from build123d import *

# Parameters (mm, degrees)
F0_R     = 11.25
F1_DEPTH = 3
F2_R     = 9.5
F3_DEPTH = 7.5
F4_R     = 3.75
F5_DEPTH = 7.5
F6_R     = 0.25
F7_DEPTH = 6
F8_SIZE2 = 0.288675
F8_SIZE  = 0.5
F9_R     = 0.3
F10_R    = 2.5


with BuildPart() as f1:
    # F0 (on Top) → F1 (new body)
    with BuildSketch(Plane.XY):
        Circle(F0_R)
    extrude(amount=F1_DEPTH)

    # F2 (on Top) → F3 (join)
    with BuildSketch(Plane.XY):
        Circle(F2_R)
    extrude(amount=F3_DEPTH)

    # F4 (on Top) → F5 (join)
    with BuildSketch(Plane.XY):
        Circle(F4_R)
    extrude(amount=-F5_DEPTH)

    # F6 (on Top) → F7 (join)
    with BuildSketch(Plane.XY):
        with Locations((0, 3.75)):
            Circle(F6_R)
        with Locations((3.75, 0)):
            Circle(F6_R)
        with Locations((0, -3.75)):
            Circle(F6_R)
        with Locations((-3.75, 0)):
            Circle(F6_R)
    extrude(amount=-F7_DEPTH)

    # F8
    f8_edges = [f1.edges().sort_by_distance(p)[0] for p in [
        (-3.75, 0, -7.5),
    ]]
    chamfer(f8_edges, length=F8_SIZE, length2=F8_SIZE2)

    # F9
    f9_edges = [f1.edges().sort_by_distance(p)[0] for p in [
        (-11.25, 0, 3),
    ]]
    fillet(f9_edges, radius=F9_R)

    # F10
    f10_edges = [f1.edges().sort_by_distance(p)[0] for p in [
        (-9.5, 0, 7.5),
    ]]
    fillet(f10_edges, radius=F10_R)


solid = f1.part
Verification items for the finished model (mm, model axes). A direction names the side the tool comes from. Coordinates: 2 decimals unless noted, no trailing zeros. Write each loop counter-clockwise with the first axis right and the second up, starting at its lowest first coordinate (ties: lowest second). Pieces come first, ordered by that corner, then holes. Notation, with made-up numbers: (-14, 53) - (22, 53) arc R24 ccw to (22, 74) - close; hole circle Ø11 at (-2.5, -7.75). An arc over 180 degrees is marked (long way). Answer as a JSON object with one key per item and string values.
(1) Mould release check, pull along Y, two halves, no side actions. Record for faces 4 (the cylindrical face through (3.464, -1.436, -3.451)), 5 (the flat face through (0, 0, -7.5)): pulls with the +Y half, pulls with the -Y half, needs draft (parallel to the pull), parting line crosses it, or undercut.
Report:
{"face 4": "parting line crosses it", "face 5": "needs draft"}
(2) Thickness scan on line 1 along Z through (x, y) = (-3.25, 9.25); line 2 along Z through (x, y) = (-1.25, 5); line 3 along X through (y, z) = (0.5, -3.75). Record the ranges inside material, lowest first.
Report:
{"line 1": "0 to 3", "line 2": "0 to 7.5", "line 3": "-3.72 to 3.72"}
(3) Tool access check on faces 1 (the flat face through (0, 10, 3)), 2 (the cylindrical face through (5.19, -9.98, 1.33)), 3 (the flat face through (-3, 3, 0)). Record the directions out of +Z, -Z, +X, -X, +Y, -Y that give a thin tool (end or side, any length) a straight path to the whole face; none if there is none.
Report:
{"face 1": "+Z", "face 2": "+Z, -Z", "face 3": "-Z"}
(4) Gauge pin test, flat ends, axial feed: pin 1 Ø1.5 at (y, z) = (5, 4.5) entering from +X; pin 2 Ø8 at (x, z) = (-4, -5.5) entering from +Y; pin 3 Ø4 at (y, z) = (-3.5, 1) entering from +X. Record the tip position at first contact, or that the pin passes through.
Report:
{"pin 1": "x = 8.5", "pin 2": "y = 4", "pin 3": "x = 11.15"}
(5) Cross-section at B-B on z = 4.25. Record the cut outline in (x, y).
Report:
{"outline": "circle Ø19 at (0, 0)"}
(6) Cross-section at A-A on z = -1.75. Record the cut outline in (x, y).
Report:
{"outline": "(-3.74, -0.25) arc R3.75 ccw to (-0.25, -3.74) arc R0.25 ccw (long way) to (0.25, -3.74) arc R3.75 ccw to (3.74, -0.25) arc R0.25 ccw (long way) to (3.74, 0.25) arc R3.75 ccw to (0.25, 3.74) arc R0.25 ccw (long way) to (-0.25, 3.74) arc R3.75 ccw to (-3.74, 0.25) arc R0.25 ccw (long way) to start"}
